CAD build for the part. Positions are in the model's coordinates, mm. A direction names the side the tool comes from. Give positions to 0.01 mm unless a question says otherwise; leave off trailing zeros. Write each loop counter-clockwise with the first axis right and the second up, starting at its lowest first coordinate (ties: lowest second). Pieces come first, ordered by that corner, then holes. Notation, with made-up numbers: M 84,52 L 131,52 A11 ccw 131,61 Z; hole C 56,30.25 d5. An arc over 180 degrees is marked long. One line per question, with ' | ' between items. Start each with the question number.
1. Wall check: L1, parallel to Z at x = 3, y = 2.75; L2, parallel to Y at x = -2, z = 14.5; L3, parallel to X at y = 1, z = 26.5. Give the ranges that are in metal, low to high.
2. Cut at C-C, the plane x = -1. Write the cut outline in (y, z).
3. Cut at B-B, the plane z = 17.5. Write the cut outline in (x, y), then the cut area to 3 significant figures.
4. Which spindle directions (+Z, -Z, +X, -X, +Y, -Y) get a long thin tool onto all of the face, cutting with end or side? Do faces 1 (the face through (-3, 3, 12.28)), 2 (the face through (-4.06, 0, 6)). Say none if no direction does.
5. Cut at A-A, the plane x = 3. Write the cut outline in (y, z), then the cut area to 3 significant figures.
```python
from build123d import *

# Parameters (mm, degrees)
SKETCH1_W           = 8.12
SKETCH1_H           = 8.12
BOSS_EXTRUDE1_DEPTH = 12.28
SKETCH2_R           = 4
BOSS_EXTRUDE2_DEPTH = 30


with BuildPart() as part:
    # Sketch1 → Boss-Extrude1 (new body)
    with BuildSketch(Plane.XY):
        Rectangle(SKETCH1_W, SKETCH1_H)
    extrude(amount=BOSS_EXTRUDE1_DEPTH)

    # Sketch2 → Boss-Extrude2 (add)
    with BuildSketch(Plane.XY):
        with Locations(Location((0, 0, 0), (0, 0, 180))):
            Circle(SKETCH2_R)
    extrude(amount=BOSS_EXTRUDE2_DEPTH)


solid = part.part
```
Here are the results:
1) L1: 0 to 12.28 | L2: -3.46 to 3.46 | L3: -3.87 to 3.87
2) outline: M -4.06,0 L 4.06,0 L 4.06,12.28 L 3.87,12.28 L 3.87,30 L -3.87,30 L -3.87,12.28 L -4.06,12.28 Z
3) outline: C 0,0 d8 | area: 50.3 mm^2
4) face 1: +Z | face 2: +Z, -Z, -X, +Y, -Y
5) outline: M -4.06,0 L 4.06,0 L 4.06,12.28 L 2.65,12.28 L 2.65,30 L -2.65,30 L -2.65,12.28 L -4.06,12.28 Z | area: 193 mm^2
